Geometry check sheet. Reference: the model listing, model coordinates, mm. Coordinates: 2 decimals unless noted, no trailing zeros. Write each loop counter-clockwise with the first axis right and the second up, starting at its lowest first coordinate (ties: lowest second). Pieces come first, ordered by that corner, then holes. Notation, with made-up numbers: (-29, 29.25) -> (-25, 29.25) arc R10 cw to (-25, 46.25) -> close; hole circle Ø3 at (-30.5, 12.25). An arc over 180 degrees is marked (long way). Answer in a Markdown table with one row per item. Add a question column.
1. Cross-section at A-A on z = 0. Record the cut outline in (x, y).
2. Cross-section at D-D on z = 15.5. Record the cut outline in (x, y).
3. Cross-section at B-B on x = 0. Record the cut outline in (y, z), and give its area (3 significant figures).
4. Mould release check, pull along Z, two halves, no side actions. Record for faces 1 (the cylindrical face through (75.49, 5.07, 20.72)), 2 (the cylindrical face through (-78.04, 4.93, -0.46)), 3 (the cylindrical face through (75.49, 5.07, -20.72)): pulls with the +Z half, pulls with the -Z half, needs draft (parallel to the pull), parting line crosses it, or undercut.
5. Cross-section at C-C on y = 3.25. Give the number of separate pieces and of enclosed holes in the cut face, and give its area (3 significant figures).
6. Scan lines: L1, parallel to Z at x = 15.5, y = 6; L2, parallel to X at y = 4.75, z = 0; L3, parallel to X at y = 1.25, z = -15. Record each from-to range of solid material in increasing order. Write a range as from..to.
7. Depth check by flat-ended pin: P1, Ø19, axis at x = 67.5, z = 0, coming from the +Y side. Enter the tip coordinate at first touch or a pass-through.
```python
from build123d import *

# Parameters (mm, degrees)
SKETCH1_W           = 160
SKETCH1_H           = 50
SKETCH1_R           = 11
SKETCH1_R_2         = 1.75
SKETCH1_R_3         = 10.55
SKETCH1_R_4         = 5
BOSS_EXTRUDE1_DEPTH = 10
FILLET1_R           = 15


with BuildPart() as part:
    # Sketch1 → Boss-Extrude1 (new body)
    with BuildSketch(Plane(origin=(0, 0, 0), x_dir=(1, 0, 0), z_dir=(0, 1, 0))):
        Rectangle(SKETCH1_W, SKETCH1_H)
        Circle(SKETCH1_R, mode=Mode.SUBTRACT)
        with Locations((15.5, 15.5)):
            Circle(SKETCH1_R_2, mode=Mode.SUBTRACT)
        with Locations((-15.5, 15.5)):
            Circle(SKETCH1_R_2, mode=Mode.SUBTRACT)
        with Locations((-15.5, -15.5)):
            Circle(SKETCH1_R_2, mode=Mode.SUBTRACT)
        with Locations((15.5, -15.5)):
            Circle(SKETCH1_R_2, mode=Mode.SUBTRACT)
        with Locations((-67.5, 0)):
            Circle(SKETCH1_R_3, mode=Mode.SUBTRACT)
        with Locations((67.5, 0)):
            Circle(SKETCH1_R_3, mode=Mode.SUBTRACT)
        with Locations((42.5, 0)):
            Circle(SKETCH1_R_4, mode=Mode.SUBTRACT)
    extrude(amount=BOSS_EXTRUDE1_DEPTH)

    # Fillet1
    fillet1_edges = [part.edges().sort_by_distance(p)[0] for p in [
        (80, 5, 25),
        (-80, 5, 25),
        (-80, 5, -25),
        (80, 5, -25),
    ]]
    fillet(fillet1_edges, radius=FILLET1_R)


solid = part.part
```
Results found:
| question | item | result |
|---|---|---|
| 1 | outline | (-80, 0) -> (-78.05, 0) -> (-78.05, 10) -> (-80, 10) -> close; (-56.95, 0) -> (-11, 0) -> (-11, 10) -> (-56.95, 10) -> close; (11, 0) -> (37.5, 0) -> (37.5, 10) -> (11, 10) -> close; (47.5, 0) -> (56.95, 0) -> (56.95, 10) -> (47.5, 10) -> close; (78.05, 0) -> (80, 0) -> (80, 10) -> (78.05, 10) -> close |
| 2 | outline | (-78.96, 0) -> (-17.25, 0) -> (-17.25, 10) -> (-78.96, 10) -> close; (-13.75, 0) -> (13.75, 0) -> (13.75, 10) -> (-13.75, 10) -> close; (17.25, 0) -> (78.96, 0) -> (78.96, 10) -> (17.25, 10) -> close |
| 3 | outline | (0, -25) -> (10, -25) -> (10, -11) -> (0, -11) -> close; (0, 11) -> (10, 11) -> (10, 25) -> (0, 25) -> close |
| 3 | area | 280 mm^2 |
| 4 | face 1 | pulls with the +Z half |
| 4 | face 2 | undercut |
| 4 | face 3 | pulls with the -Z half |
| 5 | separate pieces | 1 |
| 5 | enclosed holes | 8 |
| 5 | area | 6,610 mm^2 |
| 6 | L1 | z = -25..-17.25, -13.75..13.75, 17.25..25 |
| 6 | L2 | x = -80..-78.05, -56.95..-11, 11..37.5, 47.5..56.95, 78.05..80 |
| 6 | L3 | x = -79.14..-17.18, -13.82..13.82, 17.18..79.14 |
| 7 | P1 | passes through |
